Geometry: see drawing. Coordinates: mm, zero at the bounding-box minimum. A direction names the side the tool comes from. Give positions to 0.01 mm unless a question says otherwise; leave off trailing zeros. Loops run counter-clockwise (first coordinate to the right, second up) from the corner with the lowest first, then second, coordinate; pieces in that order, holes last. Notation, with made-up numbers: M 87.5,79.25 L 110.5,79.25 A5 cw 110.5,88.25 Z; hole C -30.75,6 d9. An arc over 180 degrees is marked long. Answer in a Markdown table with one row per item.
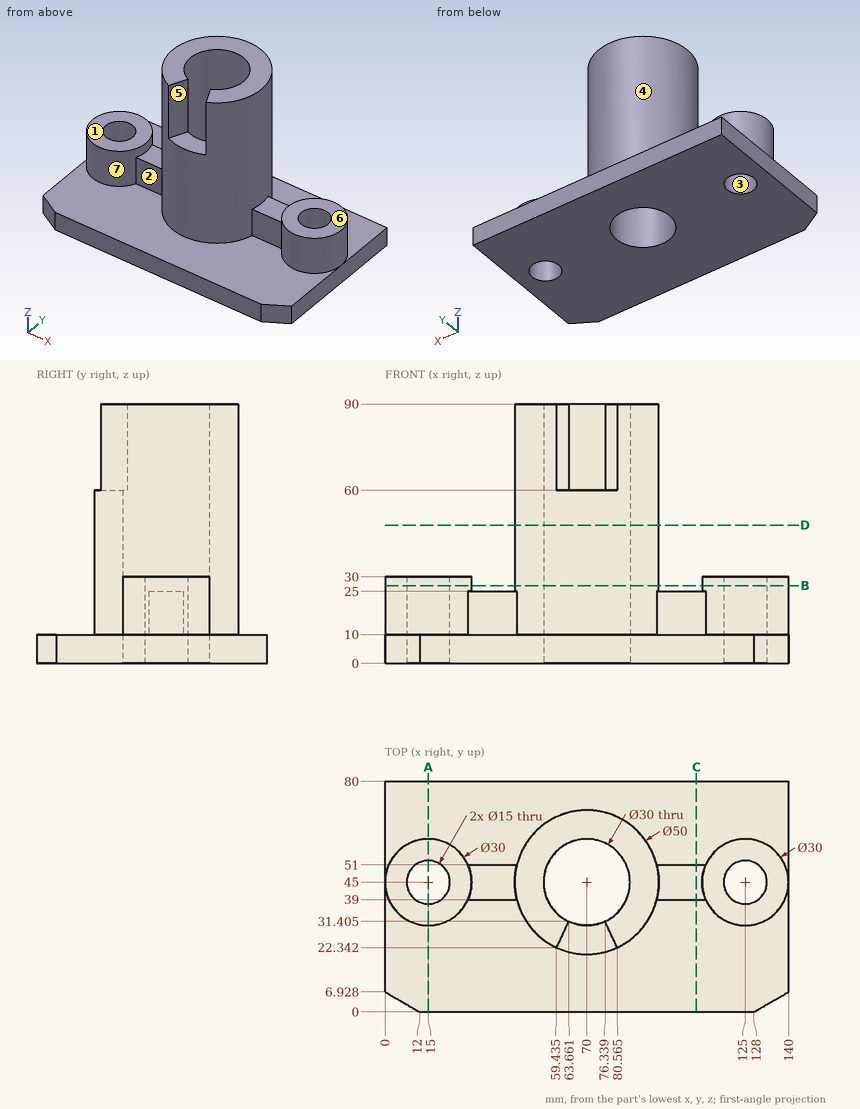
1) Pin query (flat end, axial travel): pin 1 Ø17.5 at (x, y) = (52, 66.5) entering from +Z; pin 2 Ø1 at (y, z) = (62, 51.5) entering from -X; pin 3 Ø2 at (x, z) = (32.5, 14) entering from +Y; pin 4 Ø15 at (x, y) = (17.5, 48.5) entering from +Z. Return the tip coordinate at first contact, or that it passes through.
Reply:
| item | result |
|---|---|
| pin 1 | stops at z = 90 |
| pin 2 | stops at x = 51.22 |
| pin 3 | stops at y = 51 |
| pin 4 | stops at z = 30 |
2) Pull-direction query (Y, two-part tool) for the marked faces 1, 2, 3 and 4; classes: released by +Y, released by -Y, zero draft, split by the parting line, or undercut.
Reply:
| item | result |
|---|---|
| face 1 | zero draft |
| face 2 | released by -Y |
| face 3 | undercut |
| face 4 | split by the parting line |
3) Section D-D, the plane z = 48. Return loops of the section in (x, y).
Reply:
| item | result |
|---|---|
| outline | C 70,45 d50; hole C 70,45 d30 |
4) Set-up query: the marked faces 5, 6 and 7. Return all of +Z, -Z, +X, -X, +Y, -Y with unobstructed straight access to the full face (end or side cutting, diameter ignored); none if empty.
Reply:
| item | result |
|---|---|
| face 5 | +Z, -Y |
| face 6 | +Z, +X, +Y, -Y |
| face 7 | +Z |
5) Section C-C, the plane x = 108. Return loops of the section in (y, z).
Reply:
| item | result |
|---|---|
| outline | M 0,0 L 80,0 L 80,10 L 51,10 L 51,25 L 39,25 L 39,10 L 0,10 Z |
6) Section A-A, the plane x = 15. Return loops of the section in (y, z).
Reply:
| item | result |
|---|---|
| outline | M 0,0 L 37.5,0 L 37.5,30 L 30,30 L 30,10 L 0,10 Z; M 52.5,0 L 80,0 L 80,10 L 60,10 L 60,30 L 52.5,30 Z |
7) Material intervals for L1, parallel to Y at x = 70, z = 31; L2, parallel to Z at x = 127, y = 75.5; L3, parallel to X at y = 45, z = 63, sorted ascending.
Reply:
| item | result |
|---|---|
| L1 | y = 20 to 30, 60 to 70 |
| L2 | z = 0 to 10 |
| L3 | x = 45 to 55, 85 to 95 |
8) Section B-B, the plane z = 27. Return loops of the section in (x, y).
Reply:
| item | result |
|---|---|
| outline | C 15,45 d30; C 70,45 d50; C 125,45 d30; hole C 15,45 d15; hole C 70,45 d30; hole C 125,45 d15 |
